from build123d import *

# Parameters (mm, degrees)
SKETCH_1_W          = 48
SKETCH_1_H          = 6
SKETCH_1_R          = 1.75
EXTRUDE_1_DEPTH     = 8
SKETCH_2_R          = 1.75
CUT_EXTRUDE_1_DEPTH = 45.147480109


with BuildPart() as part:
    # 草图1 → 凸台-拉伸1 (new body)
    with BuildSketch(Plane(origin=(0, 0, 0), x_dir=(1, 0, 0), z_dir=(0, 1, 0))):
        with Locations((19, 0)):
            Rectangle(SKETCH_1_W, SKETCH_1_H)
        with Locations(Location((0, 0, 0), (0, 0, 270))):
            Circle(SKETCH_1_R, mode=Mode.SUBTRACT)
        with Locations(Location((38, 0, 0), (0, 0, 270))):
            Circle(SKETCH_1_R, mode=Mode.SUBTRACT)
    extrude(amount=EXTRUDE_1_DEPTH)

    # 草图2 → 切除-拉伸1 (cut, through all)
    with BuildSketch(Plane.XY.offset(3)):
        with Locations((9, 5)):
            Circle(SKETCH_2_R)
        with Locations((29, 5)):
            Circle(SKETCH_2_R)
    extrude(amount=-CUT_EXTRUDE_1_DEPTH, mode=Mode.SUBTRACT)


solid = part.part
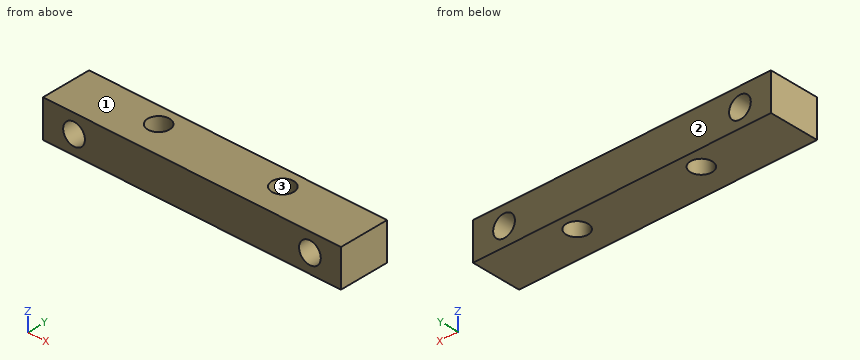
CAD build for the part. Positions are in the model's coordinates, mm. Face numbers are marked on the shaded views. Coordinates: 2 decimals unless noted, no trailing zeros. Order: outer loops, then holes, each group sorted by start corner. A loop starts at its lowest first (then second) coordinate and runs counter-clockwise, first axis right, second up.
Item 1: Band-saw the part on D-D on y = 2.25. List the corners of the cut face in (x, z).
Check sheet entries:
outline: (-5, -3) - (43, -3) - (43, 3) - (-5, 3) - close; hole circle Ø3.5 at (0, 0); hole circle Ø3.5 at (38, 0)
Item 2: Band-saw the part on C-C on y = 6.25. List the corners of the cut face in (x, z).
Check sheet entries:
outline: (-5, -3) - (7.78, -3) - (7.78, 3) - (-5, 3) - close; (10.22, -3) - (27.78, -3) - (27.78, 3) - (10.22, 3) - close; (30.22, -3) - (43, -3) - (43, 3) - (30.22, 3) - close; hole circle Ø3.5 at (0, 0); hole circle Ø3.5 at (38, 0)
Item 3: Band-saw the part on A-A on x = 29. List the corners of the cut face in (y, z), plus the area to 3 significant figures.
Check sheet entries:
outline: (0, -3) - (3.25, -3) - (3.25, 3) - (0, 3) - close; (6.75, -3) - (8, -3) - (8, 3) - (6.75, 3) - close
area: 27.0 mm2
Item 4: Drill centre lines: L1, parallel to X at y = 0.75, z = -0.15; L2, parallel to X at y = 3.5, z = -2.25; L3, parallel to X at y = 5.5, z = -0.75. Where is each one in solid material? Low to high.
Check sheet entries:
L1: x = -5 to -1.74, 1.74 to 36.26, 39.74 to 43
L2: x = -5 to 8.1, 9.9 to 28.1, 29.9 to 43
L3: x = -5 to -1.58, 1.58 to 7.32, 10.68 to 27.32, 30.68 to 36.42, 39.58 to 43
Item 5: Two-plate mould, pull along Y, no slides. Class the marked faces 1, 2 and 3: +Y half, -Y half, draft (parallel to the pull), parting line (faces both ways), or undercut.
Check sheet entries:
face 1: draft
face 2: +Y half
face 3: undercut
Item 6: Band-saw the part on B-B on z = 0. List the corners of the cut face in (x, y).
Check sheet entries:
outline: (-5, 0) - (-1.75, 0) - (-1.75, 8) - (-5, 8) - close; (1.75, 0) - (36.25, 0) - (36.25, 8) - (1.75, 8) - close; (39.75, 0) - (43, 0) - (43, 8) - (39.75, 8) - close; hole circle Ø3.5 at (9, 5); hole circle Ø3.5 at (29, 5)
